```python
from build123d import *

# Parameters (mm, degrees)
SKETCH1_W           = 100
SKETCH1_H           = 80
BOSS_EXTRUDE1_DEPTH = 2
SKETCH2_W           = 25
SKETCH2_H           = 15
BOSS_EXTRUDE2_DEPTH = 4
SKETCH3_R           = 2
CUT_EXTRUDE1_DEPTH  = 129.202964084
FILLET1_R           = 10


with BuildPart() as part:
    # Sketch1 → Boss-Extrude1 (new body)
    with BuildSketch(Plane.XY):
        with Locations((50, 40)):
            Rectangle(SKETCH1_W, SKETCH1_H)
    extrude(amount=BOSS_EXTRUDE1_DEPTH)

    # Sketch2 → Boss-Extrude2 (add)
    with BuildSketch(Plane.XY.offset(2)):
        with Locations((87.5, 41.137045181)):
            Rectangle(SKETCH2_W, SKETCH2_H)
    extrude(amount=BOSS_EXTRUDE2_DEPTH)

    # Sketch3 → Cut-Extrude1 (cut, through all)
    with BuildSketch(Plane.XY.offset(6)):
        with Locations((80.242914422, 41.137045181)):
            Circle(SKETCH3_R)
        with Locations((95.242914422, 41.137045181)):
            Circle(SKETCH3_R)
    extrude(amount=-CUT_EXTRUDE1_DEPTH, mode=Mode.SUBTRACT)

    # Fillet1
    # the kernel refuses this fillet: 10 mm, written as the material it adds along each edge
    with BuildSketch(Plane(origin=(75, 48.637045181, 2), x_dir=(0, 1, 0), z_dir=(1, 0, 0)), Plane(origin=(100, 33.637045181, 2), x_dir=(0, -1, 0), z_dir=(-1, 0, 0))) as fillet1_piece_1:
        with BuildLine():
            CenterArc((8, 10), FILLET1_R, 216.869897646, 53.130102354)
            Line((0, 4), (-0.16, 3.88))
            ThreePointArc((-0.16, 3.88), (-0.2, 2), (-0.2, 0))
            Line((-0.2, 0), (0, -0.2))
            Line((0, -0.2), (8, -0.2))
            Line((8, -0.2), (8, 0))
        make_face()
    extrude(amount=25)
    with BuildSketch(Plane(origin=(75, 33.637045181, 2), x_dir=(-1, 0, 0), z_dir=(0, 1, 0))) as fillet1_piece_2:
        with BuildLine():
            CenterArc((8, 10), FILLET1_R, 216.869897646, 53.130102354)
            Line((0, 4), (-0.16, 3.88))
            ThreePointArc((-0.16, 3.88), (-0.2, 2), (-0.2, 0))
            Line((-0.2, 0), (0, -0.2))
            Line((0, -0.2), (8, -0.2))
            Line((8, -0.2), (8, 0))
        make_face()
    extrude(amount=15)
    with BuildSketch(Plane(origin=(55, 48.637045181, 2), x_dir=(0, 1, 0), z_dir=(1, 0, 0))) as fillet1_piece_3a_section:
        with BuildLine():
            CenterArc((8, 10), FILLET1_R, 216.869897646, 53.130102354)
            Line((0, 4), (-0.16, 3.88))
            ThreePointArc((-0.16, 3.88), (-0.2, 2), (-0.2, 0))
            Line((-0.2, 0), (0, -0.2))
            Line((0, -0.2), (8, -0.2))
            Line((8, -0.2), (8, 0))
        make_face()
    fillet1_piece_3a = extrude(amount=45, mode=Mode.PRIVATE)
    fillet1_piece_3a = split(fillet1_piece_3a, bisect_by=Plane(origin=(75, 50.695879295, 3.023885124), z_dir=(-1, 0, 0)), keep=Keep.TOP, mode=Mode.PRIVATE)
    with BuildSketch(Plane(origin=(75, 33.637045181, 2), x_dir=(-1, 0, 0), z_dir=(0, 1, 0))) as fillet1_piece_3b_section:
        with BuildLine():
            CenterArc((8, 10), FILLET1_R, 216.869897646, 53.130102354)
            Line((0, 4), (-0.16, 3.88))
            ThreePointArc((-0.16, 3.88), (-0.2, 2), (-0.2, 0))
            Line((-0.2, 0), (0, -0.2))
            Line((0, -0.2), (8, -0.2))
            Line((8, -0.2), (8, 0))
        make_face()
    fillet1_piece_3b = extrude(amount=35, mode=Mode.PRIVATE)
    fillet1_piece_3b = split(fillet1_piece_3b, bisect_by=Plane(origin=(72.941165886, 48.637045181, 3.023885124), z_dir=(0, 1, 0)), keep=Keep.TOP, mode=Mode.PRIVATE)
    fillet1_piece_3 = fillet1_piece_3a & fillet1_piece_3b
    add(fillet1_piece_3)
    with BuildSketch(Plane(origin=(75, 13.637045181, 2), x_dir=(-1, 0, 0), z_dir=(0, 1, 0))) as fillet1_piece_4a_section:
        with BuildLine():
            CenterArc((8, 10), FILLET1_R, 216.869897646, 53.130102354)
            Line((0, 4), (-0.16, 3.88))
            ThreePointArc((-0.16, 3.88), (-0.2, 2), (-0.2, 0))
            Line((-0.2, 0), (0, -0.2))
            Line((0, -0.2), (8, -0.2))
            Line((8, -0.2), (8, 0))
        make_face()
    fillet1_piece_4a = extrude(amount=35, mode=Mode.PRIVATE)
    fillet1_piece_4a = split(fillet1_piece_4a, bisect_by=Plane(origin=(72.941165886, 33.637045181, 3.023885124), z_dir=(0, -1, 0)), keep=Keep.TOP, mode=Mode.PRIVATE)
    with BuildSketch(Plane(origin=(100, 33.637045181, 2), x_dir=(0, -1, 0), z_dir=(-1, 0, 0))) as fillet1_piece_4b_section:
        with BuildLine():
            CenterArc((8, 10), FILLET1_R, 216.869897646, 53.130102354)
            Line((0, 4), (-0.16, 3.88))
            ThreePointArc((-0.16, 3.88), (-0.2, 2), (-0.2, 0))
            Line((-0.2, 0), (0, -0.2))
            Line((0, -0.2), (8, -0.2))
            Line((8, -0.2), (8, 0))
        make_face()
    fillet1_piece_4b = extrude(amount=45, mode=Mode.PRIVATE)
    fillet1_piece_4b = split(fillet1_piece_4b, bisect_by=Plane(origin=(75, 31.578211067, 3.023885124), z_dir=(-1, 0, 0)), keep=Keep.TOP, mode=Mode.PRIVATE)
    fillet1_piece_4 = fillet1_piece_4a & fillet1_piece_4b
    add(fillet1_piece_4)


solid = part.part
```
The listing builds one solid part. Answer for the finished solid, in the listing's coordinates (mm). A direction names the side the tool comes from. Coordinates: 2 decimals unless noted, no trailing zeros. Loops run counter-clockwise (first coordinate to the right, second up) from the corner with the lowest first, then second, coordinate; pieces in that order, holes last. Notation, with made-up numbers: (-25.75, 21.5) - (-14.75, 21.5) arc R24 ccw to (-14.75, 32.5) - close; hole circle Ø3 at (52.25, 76.25). An arc over 180 degrees is marked (long way). Use a Markdown table: item, result. Add a question column.
1) Given pin 1 (3 mm diameter, centred on x = 95.24, y = 41.14, fed in from +Z); pin 2 (24 mm diameter, centred on x = 43, y = 29.5, fed in from +Z); pin 3 (1 mm diameter, centred on y = 43.5, z = 4, fed in from -X), each flat-ended and moving along its own axis, determine where each tip first touches the part or whether it passes through.
2) The part is cut by section A-A, the plane x = 80.5. Give the vertices of the cut face in (y, z).
3) The part is cut by section C-C, the plane y = 31. Give the vertices of the cut face in (x, z), and give its area (3 significant figures).
4) For faces 1 (the flat face through (87, 41, 6)), 2 (the flat face through (49, 41, 2)), determine the directions among +Z, -Z, +X, -X, +Y, -Y from which every point of the face is accessible in a straight line to the end or side of a thin tool.
5) The part is cut by section B-B, the plane z = 3.65. Give the vertices of the cut face in (x, y), and give its area (3 significant figures).
6) The mould has two halves that part along Y. Classify faces 3 (the flat face through (49, 0, 1)), 4 (the cylindrical face through (86.936, 52.107, 3.085)), 5 (the cylindrical face through (93.77, 42.49, 3.04)): released by +Y, released by -Y, zero draft, split by the parting line, or undercut.
7) Find the intervals of material crossed by line 1 (Z direction, x = 64, y = 33); line 2 (Y direction, x = 82, z = 1.2); line 3 (X direction, y = 50, z = 3.85), in increasing order.
8) The part is cut by section D-D, the plane x = 56. Give the vertices of the cut face in (y, z), and give its area (3 significant figures).
Here are the results:
| question | item | result |
|---|---|---|
| 1 | pin 1 | passes through |
| 1 | pin 2 | stops at z = 2 |
| 1 | pin 3 | stops at x = 72.27 |
| 2 | outline | (0, 0) - (39.15, 0) - (39.15, 6) - (33.64, 6) arc R10 cw to (25.64, 2) - (0, 2) - close; (43.12, 0) - (80, 0) - (80, 2) - (56.64, 2) arc R10 cw to (48.64, 6) - (43.12, 6) - close |
| 3 | outline | (0, 0) - (100, 0) - (100, 3.56) - (72.36, 3.56) arc R10 cw to (67, 2) - (0, 2) - close |
| 3 | area | 246 mm^2 |
| 4 | face 1 | +Z, +X, -X, +Y, -Y |
| 4 | face 2 | +Z, -X |
| 5 | outline | (72.5, 31.14) - (100, 31.14) - (100, 51.13) - (72.5, 51.13) - close; hole circle Ø4 at (80.24, 41.14); hole circle Ø4 at (95.24, 41.14) |
| 5 | area | 525 mm^2 |
| 6 | face 3 | released by -Y |
| 6 | face 4 | released by +Y |
| 6 | face 5 | undercut |
| 7 | line 1 | z = 0 to 2 |
| 7 | line 2 | y = 0 to 40.18, 42.09 to 80 |
| 7 | line 3 | x = 72.79 to 100 |
| 8 | outline | (0, 0) - (80, 0) - (80, 2) - (0, 2) - close |
| 8 | area | 160 mm^2 |
